Read the model definition and answer for the solid it produces. Units are mm, in the model's axes. A direction names the side the tool comes from. Coordinates: 2 decimals unless noted, no trailing zeros. Write each loop counter-clockwise with the first axis right and the second up, starting at its lowest first coordinate (ties: lowest second). Pieces come first, ordered by that corner, then holes. Notation, with made-up numbers: (-0.5, 63) -> (12.5, 63) arc R27 ccw to (12.5, 97) -> close; hole circle Ø6 at (-21, -29.75). An arc over 180 degrees is marked (long way). Use CSV: the item, a comma, the result in double quotes. Start each with the question number.
from build123d import *

# Parameters (mm, degrees)
SKETCH1_W           = 90
SKETCH1_H           = 90
BOSS_EXTRUDE1_DEPTH = 3
FILLET1_R           = 5
FILLET3_R           = 5
SKETCH2_R           = 10
SKETCH2_R_2         = 2
CUT_EXTRUDE1_DEPTH  = 3


with BuildPart() as part:
    # Sketch1 → Boss-Extrude1 (new body)
    with BuildSketch(Plane.XY):
        with Locations((-51.25, -17.8125)):
            Rectangle(SKETCH1_W, SKETCH1_H)
    extrude(amount=BOSS_EXTRUDE1_DEPTH)

    # Fillet1
    fillet1_edges = [part.edges().sort_by_distance(p)[0] for p in [
        (-96.25, 27.1875, 1.5),
        (-6.25, 27.1875, 1.5),
        (-6.25, -62.8125, 1.5),
        (-96.25, -62.8125, 1.5),
    ]]
    fillet(fillet1_edges, radius=FILLET1_R)

    # Fillet3
    # the kernel refuses this fillet: 5 mm, written as the material it takes off along each edge
    with BuildSketch(Plane(origin=(-91.25, 22.1875, 3), x_dir=(0, 1, 0), z_dir=(1, 0, 0))) as fillet3_piece_1:
        with BuildLine():
            CenterArc((0.417424305, -5), FILLET3_R, 23.578178478, 66.421821522)
            Line((0.417424305, 0), (0.417424305, 0.1))
            Line((0.417424305, 0.1), (5, 0.1))
            Line((5, 0.1), (5.1, 0))
            ThreePointArc((5.1, 0), (5.1, -1.5), (5.091651514, -2.96))
            Line((5.091651514, -2.96), (5, -3))
        make_face()
    revolve(axis=Axis((-91.25, 22.1875, 3), (0, 0, 1)), revolution_arc=90, mode=Mode.SUBTRACT)
    with BuildSketch(Plane(origin=(-91.25, 27.1875, 3), x_dir=(0, 0, -1), z_dir=(1, 0, 0))) as fillet3_piece_2:
        with BuildLine():
            CenterArc((5, -4.582575695), FILLET3_R, 113.578178478, 66.421821522)
            Line((0, -4.582575695), (-0.1, -4.582575695))
            Line((-0.1, -4.582575695), (-0.1, 0))
            Line((-0.1, 0), (0, 0.1))
            ThreePointArc((0, 0.1), (1.5, 0.1), (2.96, 0.091651514))
            Line((2.96, 0.091651514), (3, 0))
        make_face()
    extrude(amount=80, mode=Mode.SUBTRACT)
    with BuildSketch(Plane(origin=(-11.25, 22.1875, 3), x_dir=(0, 1, 0), z_dir=(-1, 0, 0))) as fillet3_piece_3:
        with BuildLine():
            CenterArc((0.417424305, 5), FILLET3_R, 270, 66.421821522)
            Line((0.417424305, 0), (0.417424305, -0.1))
            Line((0.417424305, -0.1), (5, -0.1))
            Line((5, -0.1), (5.1, 0))
            ThreePointArc((5.1, 0), (5.1, 1.5), (5.091651514, 2.96))
            Line((5.091651514, 2.96), (5, 3))
        make_face()
    revolve(axis=Axis((-11.25, 22.1875, 3), (0, 0, -1)), revolution_arc=90, mode=Mode.SUBTRACT)
    with BuildSketch(Plane(origin=(-6.25, 22.1875, 3), x_dir=(-1, 0, 0), z_dir=(0, -1, 0)), Plane(origin=(-11.25, -62.8125, 3), x_dir=(0, 1, 0), z_dir=(-1, 0, 0)), Plane(origin=(-96.25, -57.8125, 3), x_dir=(1, 0, 0), z_dir=(0, 1, 0))) as fillet3_piece_4:
        with BuildLine():
            CenterArc((4.582575695, 5), FILLET3_R, 203.578178478, 66.421821522)
            Line((0, 3), (-0.091651514, 2.96))
            ThreePointArc((-0.091651514, 2.96), (-0.1, 1.5), (-0.1, 0))
            Line((-0.1, 0), (0, -0.1))
            Line((0, -0.1), (4.582575695, -0.1))
            Line((4.582575695, -0.1), (4.582575695, 0))
        make_face()
    extrude(amount=80, mode=Mode.SUBTRACT)
    with BuildSketch(Plane(origin=(-11.25, -57.8125, 3), x_dir=(1, 0, 0), z_dir=(0, 1, 0))) as fillet3_piece_5:
        with BuildLine():
            CenterArc((0.417424305, 5), FILLET3_R, 270, 66.421821522)
            Line((5, 3), (5.091651514, 2.96))
            ThreePointArc((5.091651514, 2.96), (5.1, 1.5), (5.1, 0))
            Line((5.1, 0), (5, -0.1))
            Line((5, -0.1), (0.417424305, -0.1))
            Line((0.417424305, -0.1), (0.417424305, 0))
        make_face()
    revolve(axis=Axis((-11.25, -57.8125, 3), (0, 0, -1)), revolution_arc=90, mode=Mode.SUBTRACT)
    with BuildSketch(Plane(origin=(-91.25, -57.8125, 3), x_dir=(0, -1, 0), z_dir=(1, 0, 0))) as fillet3_piece_6:
        with BuildLine():
            CenterArc((0.417424305, 5), FILLET3_R, 270, 66.421821522)
            Line((5, 3), (5.091651514, 2.96))
            ThreePointArc((5.091651514, 2.96), (5.1, 1.5), (5.1, 0))
            Line((5.1, 0), (5, -0.1))
            Line((5, -0.1), (0.417424305, -0.1))
            Line((0.417424305, -0.1), (0.417424305, 0))
        make_face()
    revolve(axis=Axis((-91.25, -57.8125, 3), (0, 0, -1)), revolution_arc=90, mode=Mode.SUBTRACT)

    # Sketch2 → Cut-Extrude1 (cut)
    with BuildSketch(Plane.XY.offset(3)):
        with Locations((-51.491961851, -15.545023704)):
            Circle(SKETCH2_R)
        with Locations((-88.238370767, -19.051344954)):
            Circle(SKETCH2_R_2)
        with Locations((-14.261629233, -19.051344954)):
            Circle(SKETCH2_R_2)
        with BuildLine():
            Line((-54.583479712, -29.628619656), (-47.996622456, -29.628619656))
            ThreePointArc((-47.996622456, -29.628619656), (-45.496622456, -32.128619656), (-47.996622456, -34.628619656))
            Line((-47.996622456, -34.628619656), (-54.583479712, -34.628619656))
            ThreePointArc((-54.583479712, -34.628619656), (-57.083479712, -32.128619656), (-54.583479712, -29.628619656))
        make_face()
        with BuildLine():
            Line((-53.113614206, 0.771303592), (-49.397460357, 0.771303592))
            ThreePointArc((-49.397460357, 0.771303592), (-48.397460357, -0.228696408), (-49.397460357, -1.228696408))
            Line((-49.397460357, -1.228696408), (-53.113614206, -1.228696408))
            ThreePointArc((-53.113614206, -1.228696408), (-54.113614206, -0.228696408), (-53.113614206, 0.771303592))
        make_face()
    extrude(amount=-CUT_EXTRUDE1_DEPTH, mode=Mode.SUBTRACT)


solid = part.part
1) Which of the six approach directions +Z, -Z, +X, -X, +Y, -Y give full straight-line access (tool end or side, diameter ignored) to faces 5 (the face through (-51, -1.229, 2)), 6 (the face through (-94.44, -18.37, 2.16))?
2) Each of these flat-tipped pins is pushed along its axis until it touches: pin 1 (1 mm diameter, centred on y = 5, z = 1, fed in from -X); pin 2 (0.9 mm diameter, centred on x = -50.5, z = 2, fed in from -Y); pin 3 (1.5 mm diameter, centred on x = -50.5, z = 1.5, fed in from -Y). Where does it stop, or does it pass through?
3) Section D-D, the plane z = 2.25 is taken. Count the separate pieces of the cut face and the enclosed holes in it, plus the area to 3 significant figures.
4) Section A-A, the plane y = -12.5 is taken. Give the vertices of the cut face in (x, z), plus the area to 3 significant figures.
5) Section C-C, the plane x = -65.5 is taken. Give the vertices of the cut face in (y, z).
6) Section B-B, the plane x = -43 is taken. Give the vertices of the cut face in (y, z), plus the area to 3 significant figures.
7) The mould has two halves that part along Y. Classify faces 1 (the face through (-51.81, 25.38, 2.16)), 2 (the face through (-50.69, -61.002, 2.161)), 3 (the face through (-62, -17, 0)), 4 (the face through (-54.113, -0.251, 1.521)): pulls with the +Y half, pulls with the -Y half, needs draft (parallel to the pull), parting line crosses it, or undercut.
8) Find the intervals of material crossed by line 1 along Y through (x, z) = (-47.5, 0.4); line 2 along X through (y, z) = (-34, 1.5); line 3 along X through (y, z) = (-22, 0.5), in increasing order.
The answers:
1,face 5,"+Z, -Z"
1,face 6,"+Z, -X, +Y, -Y"
2,pin 1,"stops at x = -96"
2,pin 2,"stops at y = -61.75"
2,pin 3,"stops at y = -62.41"
3,separate pieces,"1"
3,enclosed holes,"5"
3,area,"7,000 mm^2"
4,outline,"(-96.25, 0) -> (-61.02, 0) -> (-61.02, 3) -> (-91.67, 3) arc R5 ccw to start; (-41.97, 0) -> (-6.25, 0) arc R5 ccw to (-10.83, 3) -> (-41.97, 3) -> close"
4,area,"205 mm^2"
5,outline,"(-62.81, 0) -> (27.19, 0) arc R5 ccw to (22.6, 3) -> (-58.23, 3) arc R5 ccw to start"
6,outline,"(-62.81, 0) -> (-20.83, 0) -> (-20.83, 3) -> (-58.23, 3) arc R5 ccw to start; (-10.26, 0) -> (27.19, 0) arc R5 ccw to (22.6, 3) -> (-10.26, 3) -> close"
6,area,"231 mm^2"
7,face 1,"pulls with the +Y half"
7,face 2,"pulls with the -Y half"
7,face 3,"needs draft"
7,face 4,"undercut"
8,line 1,"y = -62.62 to -34.58, -29.68 to -24.71, -6.38 to 26.99"
8,line 2,"x = -95.24 to -56.24, -46.34 to -7.26"
8,line 3,"x = -96 to -59.13, -43.85 to -6.5"
